Read the model definition and answer for the solid it produces. Units are mm, in the model's axes. A direction names the side the tool comes from. Give positions to 0.01 mm unless a question says otherwise; leave off trailing zeros. Order: outer loops, then holes, each group sorted by start corner. A loop starts at its lowest first (then second) coordinate and runs counter-clockwise, first axis right, second up.
```python
from build123d import *

# Parameters (mm, degrees)
SKETCH1_W           = 120
SKETCH1_H           = 25
BOSS_EXTRUDE1_DEPTH = 3


with BuildPart() as part:
    # Sketch1 → Boss-Extrude1 (new body)
    with BuildSketch(Plane(origin=(0, 0, 0), x_dir=(1, 0, 0), z_dir=(0, 1, 0))):
        with Locations((33.666007905, 0)):
            Rectangle(SKETCH1_W, SKETCH1_H)
        Polygon((-23.333992095, -7.72447191), (-23.333992095, 9.5), (3.862542499, 9.5), align=None, mode=Mode.SUBTRACT)
        Polygon((90.666007905, -7.72447191), (90.666007905, 9.5), (63.469473311, 9.5), align=None, mode=Mode.SUBTRACT)
        Polygon((-20.530526689, -9.5), (31.059548849, -9.5), (6.622144647, 7.696691846), align=None, mode=Mode.SUBTRACT)
        Polygon((60.709871163, 7.696691846), (36.272466961, -9.5), (87.862542499, -9.5), align=None, mode=Mode.SUBTRACT)
        Polygon((9.272466961, 9.5), (58.059548849, 9.5), (33.666007905, -7.665825109), align=None, mode=Mode.SUBTRACT)
    extrude(amount=BOSS_EXTRUDE1_DEPTH)


solid = part.part
```
1) For a pull along Z with two mould halves and no side action, classify faces 3 (the face through (33, 1, 12.5)), 4 (the face through (21.64, 1.479, -0.797)), 5 (the face through (38, 0, 6)) as released by +Z, released by -Z, zero draft, split by the parting line, or undercut.
Final values:
face 3: released by +Z
face 4: undercut
face 5: zero draft
2) A tool of negligible diameter and unlimited length cuts with its end or side. For faces 1 (the face through (19.01, 1.48, 1.02)), 2 (the face through (33, 1, -12.5)), from which of +Z, -Z, +X, -X, +Y, -Y can it reach the whole face along a straight path? Write none if from no direction.
Final values:
face 1: +Y, -Y
face 2: -Z, +X, -X, +Y, -Y
3) Consider L1, parallel to X at y = 0.7, z = -4; L2, parallel to X at y = 1.6, z = 5.5; L3, parallel to Z at x = -6, y = 0.7. Determine where each line is inside the solid, lowest interval first.
Final values:
L1: x = -26.33 to -23.33, -4.82 to 0.79, 11.88 to 17.09, 50.24 to 55.46, 66.55 to 72.15, 90.67 to 93.67
L2: x = -26.33 to -23.33, -19.82 to -14.21, 25.38 to 30.59, 36.74 to 41.96, 81.55 to 87.15, 90.67 to 93.67
L3: z = -12.5 to -9.5, -3.25 to 0.3, 9.5 to 12.5
4) The part is cut by section D-D on x = 40. Determine the outline of the cut face in (y, z).
Final values:
outline: (0, -12.5) - (3, -12.5) - (3, -9.5) - (0, -9.5) - close; (0, 3.21) - (3, 3.21) - (3, 6.88) - (0, 6.88) - close; (0, 9.5) - (3, 9.5) - (3, 12.5) - (0, 12.5) - close
5) The part is cut by section B-B on z = -5.25. Determine the outline of the cut face in (x, y).
Final values:
outline: (-26.33, 0) - (-23.33, 0) - (-23.33, 3) - (-26.33, 3) - close; (-2.85, 0) - (2.76, 0) - (2.76, 3) - (-2.85, 3) - close; (10.1, 0) - (15.31, 0) - (15.31, 3) - (10.1, 3) - close; (52.02, 0) - (57.23, 0) - (57.23, 3) - (52.02, 3) - close; (64.57, 0) - (70.18, 0) - (70.18, 3) - (64.57, 3) - close; (90.67, 0) - (93.67, 0) - (93.67, 3) - (90.67, 3) - close
6) The part is cut by section A-A on y = 1.45. Determine the outline of the cut face in (x, z), and give its area (3 significant figures).
Final values:
outline: (-26.33, -12.5) - (93.67, -12.5) - (93.67, 12.5) - (-26.33, 12.5) - close; hole (-23.33, -9.5) - (3.86, -9.5) - (-23.33, 7.72) - close; hole (-20.53, 9.5) - (6.62, -7.7) - (31.06, 9.5) - close; hole (9.27, -9.5) - (58.06, -9.5) - (33.67, 7.67) - close; hole (36.27, 9.5) - (60.71, -7.7) - (87.86, 9.5) - close; hole (63.47, -9.5) - (90.67, -9.5) - (90.67, 7.72) - close
area: 1,230 mm2
7) The part is cut by section C-C on x = 66. Determine the outline of the cut face in (y, z), and give its area (3 significant figures).
Final values:
outline: (0, -12.5) - (3, -12.5) - (3, -9.5) - (0, -9.5) - close; (0, -7.9) - (3, -7.9) - (3, -4.35) - (0, -4.35) - close; (0, 9.5) - (3, 9.5) - (3, 12.5) - (0, 12.5) - close
area: 28.7 mm2
8) Given pin 1 (4 mm diameter, centred on x = 31.5, z = 3.5, fed in from -Y), flat-ended and moving along its own axis, determine where the tip first touches the part or whether it passes through.
Final values:
pin 1: passes through
